The model under review builds one solid part; all positions refer to its coordinate system, in mm. A direction names the side the tool comes from. Coordinates: 2 decimals unless noted, no trailing zeros. Write each loop counter-clockwise with the first axis right and the second up, starting at its lowest first coordinate (ties: lowest second). Pieces come first, ordered by that corner, then holes.
```python
from build123d import *

# Parameters (mm, degrees)
F0_R     = 3.5687
F1_DEPTH = 2.54
F2_R     = 2.2352
F3_DEPTH = 2.54
F4_W     = 1.5494
F4_H     = 32.8676
F5_DEPTH = 3.5687
F6_R     = 0.889
F7_DEPTH = 25.4


with BuildPart() as f1:
    # F0 (on Right) → F1 (new body)
    with BuildSketch(Plane.YZ):
        Circle(F0_R)
    extrude(amount=F1_DEPTH)

    # F2 (on face) → F3 (cut)
    with BuildSketch(Plane.YZ.offset(2.54)):
        Circle(F2_R)
    extrude(amount=-F3_DEPTH, mode=Mode.SUBTRACT)

    # F4 (on Front) → F5 (join, symmetric)
    with BuildSketch(Plane.XZ):
        with Locations((-0.7747, 0)):
            Rectangle(F4_W, F4_H)
    extrude(amount=F5_DEPTH, both=True)

    # F6 (on face) → F7 (cut)
    with BuildSketch(Plane(origin=(-1.5494, 0, 0), x_dir=(0, -1, 0), z_dir=(-1, 0, 0))):
        with Locations((0, -10.668)):
            Circle(F6_R)
        with Locations((0, 10.668)):
            Circle(F6_R)
    extrude(amount=-F7_DEPTH, mode=Mode.SUBTRACT)


solid = f1.part
```
Item 1: To check wall thickness, follow line 1 along Z through (x, y) = (-0.85, 0); line 2 along Z through (x, y) = (1.8, 0); line 3 along X through (y, z) = (3.25, -14.5). State the ranges of each line that lie inside material, in increasing order.
Solved:
line 1: z = -16.43 to -11.56, -9.78 to 9.78, 11.56 to 16.43
line 2: z = -3.57 to -2.24, 2.24 to 3.57
line 3: x = -1.55 to 0
Item 2: Mouldability with a two-part tool opening along Y and no side actions: class faces 1 (the face through (1.252, -3.565, 0.157)), 2 (the face through (-0.8, 0.2, 9.8)), 3 (the face through (0, -1, -10)), 4 (the face through (1, -2, -1)) as pulls with the +Y half, pulls with the -Y half, needs draft (parallel to the pull), parting line crosses it, or undercut.
Solved:
face 1: parting line crosses it
face 2: undercut
face 3: needs draft
face 4: undercut
Item 3: Machinability: for faces 5 (the face through (-1, -3.569, 0)), 6 (the face through (0, 0, 0)), which of the approach directions +Z, -Z, +X, -X, +Y, -Y give a long, thin tool a straight path to every point of the face, cutting with its end or side? Answer none if there is none.
Solved:
face 5: +Z, -Z, +X, -X, -Y
face 6: +X
Item 4: Take a section at D-D, the plane y = 1.75. Write out the cut boundary in (x, z), plus the area to 3 significant figures.
Solved:
outline: (-1.55, -16.43) - (0, -16.43) - (0, -3.11) - (2.54, -3.11) - (2.54, -1.39) - (0, -1.39) - (0, 1.39) - (2.54, 1.39) - (2.54, 3.11) - (0, 3.11) - (0, 16.43) - (-1.55, 16.43) - close
area: 59.7 mm2
Item 5: For pin 1 (2.5 mm diameter, centred on y = 0, z = -10.668, fed in from +X), flat-tipped, find the tip position at first contact; note if it passes through.
Solved:
pin 1: stops at x = 0
Item 6: Take a section at A-A, the plane y = 0. Write out the cut boundary in (x, z), plus the area to 3 significant figures.
Solved:
outline: (-1.55, -16.43) - (0, -16.43) - (0, -11.56) - (-1.55, -11.56) - close; (-1.55, -9.78) - (0, -9.78) - (0, -3.57) - (2.54, -3.57) - (2.54, -2.24) - (0, -2.24) - (0, 2.24) - (2.54, 2.24) - (2.54, 3.57) - (0, 3.57) - (0, 9.78) - (-1.55, 9.78) - close; (-1.55, 11.56) - (0, 11.56) - (0, 16.43) - (-1.55, 16.43) - close
area: 52.2 mm2
Item 7: Take a section at B-B, the plane z = 11. Write out the cut boundary in (x, y).
Solved:
outline: (-1.55, -3.57) - (0, -3.57) - (0, -0.82) - (-1.55, -0.82) - close; (-1.55, 0.82) - (0, 0.82) - (0, 3.57) - (-1.55, 3.57) - close
Item 8: Take a section at C-C, the plane x = 1.95. Write out the cut boundary in (y, z), plus the area to 3 significant figures.
Solved:
outline: circle Ø7.14 at (0, 0); hole circle Ø4.47 at (0, 0)
area: 24.3 mm2
